```python
from build123d import *

# Parameters (mm, degrees)
F0_R     = 1.75
F1_DEPTH = 1.6
F2_R     = 1


with BuildPart() as f1:
    # F0 (on Top) → F1 (new body)
    with BuildSketch(Plane.XY):
        Polygon((20, 21), (-20, 21), (-20, -21), (-4, -21), (-4, -14), (20, -14), align=None)
        with Locations((-15.75, -16)):
            Circle(F0_R, mode=Mode.SUBTRACT)
        with Locations((15.75, -2)):
            Circle(F0_R, mode=Mode.SUBTRACT)
        with Locations((-15.75, 2)):
            Circle(F0_R, mode=Mode.SUBTRACT)
        with Locations((15.75, 16)):
            Circle(F0_R, mode=Mode.SUBTRACT)
    extrude(amount=F1_DEPTH)

    # F2
    f2_edges = [f1.edges().sort_by_distance(p)[0] for p in [
        (-20, -21, 0.8),
        (20, 21, 0.8),
        (-20, 21, 0.8),
        (-4, -14, 0.8),
        (-4, -21, 0.8),
        (20, -14, 0.8),
    ]]
    fillet(f2_edges, radius=F2_R)


solid = f1.part
```
The listing builds one solid part. Answer for the finished solid, in the listing's coordinates (mm). A direction names the side the tool comes from. Coordinates: 2 decimals unless noted, no trailing zeros. Loops run counter-clockwise (first coordinate to the right, second up) from the corner with the lowest first, then second, coordinate; pieces in that order, holes last. Notation, with made-up numbers: (79.25, 50.5) - (130.25, 50.5) arc R16 ccw to (130.25, 80.5) - close; hole circle Ø7 at (77.5, 24.5). An arc over 180 degrees is marked (long way). Write item = value, one per line.
1) This flat-tipped pin is pushed along its axis until it touches: P1, Ø3, axis at x = -15.75, y = -16, coming from the -Z side. Where does it stop, or does it pass through?
Responses:
P1 = through
2) Section A-A (y = 16) is taken. Determine the outline of the cut face in (x, z), plus the area to 3 significant figures.
Responses:
outline = (-20, 0) - (14, 0) - (14, 1.6) - (-20, 1.6) - close; (17.5, 0) - (20, 0) - (20, 1.6) - (17.5, 1.6) - close
area = 58.4 mm^2
3) Section B-B (x = -15.75) is taken. Determine the outline of the cut face in (y, z), plus the area to 3 significant figures.
Responses:
outline = (-21, 0) - (-17.75, 0) - (-17.75, 1.6) - (-21, 1.6) - close; (-14.25, 0) - (0.25, 0) - (0.25, 1.6) - (-14.25, 1.6) - close; (3.75, 0) - (21, 0) - (21, 1.6) - (3.75, 1.6) - close
area = 56.0 mm^2
4) Determine the mould class of faces 3 (the face through (19.699, 20.715, 0.811)), 4 (the face through (20, 3, 1)), 5 (the face through (15.522, 17.735, 0.789)) for opening direction Y: pulls with the +Y half, pulls with the -Y half, needs draft (parallel to the pull), parting line crosses it, or undercut.
Responses:
face_3 = pulls with the +Y half
face_4 = needs draft
face_5 = undercut
5) Section C-C (z = 0.6) is taken. Determine the outline of the cut face in (x, y).
Responses:
outline = (-20, -20) arc R1 ccw to (-19, -21) - (-5, -21) arc R1 ccw to (-4, -20) - (-4, -15) arc R1 cw to (-3, -14) - (19, -14) arc R1 ccw to (20, -13) - (20, 20) arc R1 ccw to (19, 21) - (-19, 21) arc R1 ccw to (-20, 20) - close; hole circle Ø3.5 at (-15.75, -16); hole circle Ø3.5 at (-15.75, 2); hole circle Ø3.5 at (15.75, -2); hole circle Ø3.5 at (15.75, 16)
6) Section D-D (y = -16) is taken. Determine the outline of the cut face in (x, z), plus the area to 3 significant figures.
Responses:
outline = (-20, 0) - (-17.5, 0) - (-17.5, 1.6) - (-20, 1.6) - close; (-14, 0) - (-4, 0) - (-4, 1.6) - (-14, 1.6) - close
area = 20.0 mm^2
7) Which of the six approach directions +Z, -Z, +X, -X, +Y, -Y give full straight-line access (tool end or side, diameter ignored) to faces 1 (the face through (8, -14, 1)), 2 (the face through (0, 0, 0))?
Responses:
face_1 = +Z, -Z, +X, -Y
face_2 = -Z, +X, -X, +Y, -Y
8) Find the intervals of material crossed by line 1 along Y through (x, z) = (15.75, 0.8); line 2 along Y through (x, z) = (-15.75, 1.35); line 3 along Y through (x, z) = (8, 1.4), in increasing order.
Responses:
line_1 = -14 to -3.75, -0.25 to 14.25, 17.75 to 21
line_2 = -21 to -17.75, -14.25 to 0.25, 3.75 to 21
line_3 = -14 to 21
